```python
from build123d import *

# Parameters (mm, degrees)
F1_DEPTH = 15
F2_R     = 7
F3_R     = 3
F4_DEPTH = 25
F5_SIZE2 = 1
F5_SIZE  = 1


with BuildPart() as f1:
    # F0 (on Top) → F1 (new body)
    with BuildSketch(Plane.XY):
        with BuildLine():
            ThreePointArc((-2, 20.105969), (-2.453959, 18.837208), (-3.609756, 18.144411))
            ThreePointArc((-3.609756, 18.144411), (0, -18.5), (3.609756, 18.144411))
            ThreePointArc((3.609756, 18.144411), (2.453959, 18.837208), (2, 20.105969))
            Line((2, 20.105969), (2, 33))
            Line((2, 33), (0.5, 33))
            Line((0.5, 33), (0.5, 16.992645))
            ThreePointArc((0.5, 16.992645), (0, -17), (-0.5, 16.992645))
            Line((-0.5, 16.992645), (-0.5, 33))
            Line((-0.5, 33), (-2, 33))
            Line((-2, 33), (-2, 20.105969))
        make_face()
    extrude(amount=F1_DEPTH)

    # F2
    f2_edges = [f1.edges().sort_by_distance(p)[0] for p in [
        (1.25, 33, 15),
        (-1.25, 33, 15),
        (1.25, 33, 0),
        (-1.25, 33, 0),
    ]]
    fillet(f2_edges, radius=F2_R)

    # F3 (on face) → F4 (cut)
    with BuildSketch(Plane.YZ.offset(2)):
        with Locations((26, 7.5)):
            Circle(F3_R)
    extrude(amount=-F4_DEPTH, mode=Mode.SUBTRACT)

    # F5
    f5_edges = [f1.edges().sort_by_distance(p)[0] for p in [
        (2, 23.052985, 15),
    ]]
    chamfer(f5_edges, length=F5_SIZE, length2=F5_SIZE2)


solid = f1.part
```
For this review, take the finished solid that the model builds, in its own axes (mm). A direction names the side the tool comes from. Round coordinates to 2 decimals unless told otherwise and drop trailing zeros. Write each loop counter-clockwise with the first axis right and the second up, starting at its lowest first coordinate (ties: lowest second). Pieces come first, ordered by that corner, then holes. Notation, with made-up numbers: (15, 24) - (20, 24) arc R17 cw to (20, 52) - close; hole circle Ø3 at (78.25, -34). An arc over 180 degrees is marked (long way). Use CSV: the item, a comma, the result in double quotes.
1) Wall thickness on line 1 along X through (y, z) = (21, 10.5); line 2 along X through (y, z) = (0, 6.5); line 3 along Y through (x, z) = (5.5, 9.75): over which ranges is each line inside the solid? List them lowest first. Write a range as from..to.
Conclusion:
line 1,"x = -2..-0.5, 0.5..2"
line 2,"x = -18.5..-17, 17..18.5"
line 3,"y = -17.66..-16.09, 16.09..17.66"
2) Clearance check with flat-ended pins moving along their axes: pin 1 Ø1 at (x, z) = (-11.5, 8) entering from -Y; pin 2 Ø3.5 at (y, z) = (28.5, 6) entering from -X; pin 3 Ø4.5 at (y, z) = (22, 9.5) entering from +X. State where each tip first meets the part, or that it passes through.
Conclusion:
pin 1,"stops at y = -14.87"
pin 2,"stops at x = -2"
pin 3,"stops at x = 2.03"
3) The part is to be moulded in two halves that separate along Y. For faces 6 (the cylindrical face through (-0.8, 31, 12.9)), 7 (the flat face through (-2, 24.8, 4.5)), 8 (the cylindrical face through (1.3, 23, 7.6)), say which applies: pulls with the +Y half, pulls with the -Y half, needs draft (parallel to the pull), parting line crosses it, or undercut.
Conclusion:
face 6,"pulls with the +Y half"
face 7,"needs draft"
face 8,"undercut"
4) For faces 1 (the flat face through (2, 23, 6)), 2 (the flat face through (1.5, 23.1, 0.5)), 3 (the flat face through (1.5, 23, 14.5)), 4 (the flat face through (-1.5, 23, 0.5)), 5 (the flat face through (0.5, 23, 9)), list the 3-axis set-ups (+Z, -Z, +X, -X, +Y, -Y) from which the entire face can be reached by the end or side of a thin tool; tool diameter is ignored.
Conclusion:
face 1,"+Z, -Z, +X, +Y"
face 2,"-Z, +X, +Y"
face 3,"+Z, +X, +Y"
face 4,"-Z, -X, +Y"
face 5,"+Z, -Z, +Y"
5) Add section B-B on z = 9.25. Count the separate pieces of the cut face and the enclosed holes in it, and give its area (3 significant figures).
Conclusion:
separate pieces,"3"
enclosed holes,"0"
area,"195 mm^2"
6) Add section A-A on y = 21. Write out the cut boundary in (x, z).
Conclusion:
outline,"(-2, 1) - (-1, 0) - (-0.5, 0) - (-0.5, 15) - (-1, 15) - (-2, 14) - close; (0.5, 0) - (1, 0) - (2, 1) - (2, 14) - (1, 15) - (0.5, 15) - close"
